```python
from build123d import *

# Parameters (mm, degrees)
F0_W      = 50.8
F0_H      = 50.8
F1_DEPTH  = 406.4
F1_FACE_W = 50.8
F1_FACE_H = 406.4
F2_DEPTH  = 31.75
F3_R      = 7.9375
F4_DEPTH  = 19.05


with BuildPart() as f1:
    # F0 (on Top) → F1 (new body)
    with BuildSketch(Plane.XY):
        with Locations((-62.744076, -41.949181)):
            Rectangle(F0_W, F0_H)
    extrude(amount=F1_DEPTH)

    # F1_face (on face) → F2 (cut)
    with BuildSketch(Plane(origin=(-37.344076, -41.949181, 203.2), x_dir=(0, 1, 0), z_dir=(1, 0, 0))):
        Rectangle(F1_FACE_W, F1_FACE_H)
    extrude(amount=-F2_DEPTH, mode=Mode.SUBTRACT)

    # F3 (on face) → F4 (cut)
    with BuildSketch(Plane(origin=(-88.144076, 0, 0), x_dir=(0, -1, 0), z_dir=(-1, 0, 0))):
        with Locations((41.949181, 84.1375)):
            Circle(F3_R)
    extrude(amount=-F4_DEPTH, mode=Mode.SUBTRACT)


solid = f1.part
```
Can you work these out from the model? Positions are in its coordinate system, mm. Round coordinates to 2 decimals unless told otherwise and drop trailing zeros. Order: outer loops, then holes, each group sorted by start corner. A loop starts at its lowest first (then second) coordinate and runs counter-clockwise, first axis right, second up.
(1) If I drill on L1, parallel to Z at x = -83.5, y = -41; L2, parallel to Z at x = -79, y = -37.5; L3, parallel to Y at x = -85.25, z = 87, over which ranges is the centre line in solid material (lowest first)?
Results are:
L1: z = 0 to 76.26, 92.02 to 406.4
L2: z = 0 to 77.56, 90.71 to 406.4
L3: y = -67.35 to -49.35, -34.55 to -16.55
(2) If we section it at A-A (y = -41.5): Please give me the cut outline in (x, z).
Results are:
outline: (-88.14, 0) - (-69.09, 0) - (-69.09, 76.21) - (-88.14, 76.21) - close; (-88.14, 92.06) - (-69.09, 92.06) - (-69.09, 406.4) - (-88.14, 406.4) - close
(3) We'd pull the mould along Y, two halves only. Please class faces 1 (the face through (-79, -42, 406.4)), 2 (the face through (-78.75, -40.92, 92.01)), 3 (the face through (-79, -16.549, 200)), 4 (the face through (-79, -67.349, 200)): +Y half, -Y half, draft (parallel to the pull), parting line (faces both ways), or undercut.
Results are:
face 1: draft
face 2: undercut
face 3: +Y half
face 4: -Y half
